Geometry: final body of the model. Coordinates: model frame, mm. Round coordinates to 2 decimals unless told otherwise and drop trailing zeros. Write each loop counter-clockwise with the first axis right and the second up, starting at its lowest first coordinate (ties: lowest second). Pieces come first, ordered by that corner, then holes. Notation, with made-up numbers: M 62,38 L 94,38 A31 ccw 94,77 Z; hole C 66,77.25 d5. An arc over 180 degrees is marked long. Use one line per item in the form item = value. Start each with the question number.
Item 1: Pin query (flat end, axial travel): pin 1 Ø5.5 at (x, z) = (46.4, 123.19) entering from +Y; pin 2 Ø7.5 at (x, z) = (102.32, 78.74) entering from +Y. Return the tip coordinate at first contact, or that it passes through.
Item 2: Ray query, probe 1 along X at (y, z) = (5.5, 123.19) (3 decimals); probe 2 along X at (y, z) = (4.25, -37.5) (3 decimals); probe 3 along X at (y, z) = (3, 78.74) (3 decimals). Return the intervals inside material, ascending.
Item 3: Section query A-A (z = 78.74). Return loops of the section in (x, y) (3 decimals).
Item 4: Section query D-D (z = 123.19). Return loops of the section in (x, y) (3 decimals), and give its area (3 significant figures).
Item 5: Section query B-B (x = 0). Return loops of the section in (y, z).
Item 6: Pull-direction query (X, two-part tool) for faces 1 (the cylindrical face through (100.39, 6.26, 76.22)), 2 (the flat face through (210.274, 6, 47)), 3 (the flat face through (44, 6, -50.8)), 4 (the flat face through (-117.475, 6, 47)); classes: pulls with the +X half, pulls with the -X half, needs draft (parallel to the pull), parting line crosses it, or undercut.
Item 7: Section query C-C (z = -38.1). Return loops of the section in (x, y) (3 decimals), and give its area (3 significant figures).
from build123d import *

# Parameters (mm, degrees)
SKETCH1_W           = 327.74935392
SKETCH1_H           = 193.04
SKETCH1_R           = 14.2875
SKETCH1_R_2         = 3.175
BOSS_EXTRUDE1_DEPTH = 12.7


with BuildPart() as part:
    # Sketch1 → Boss-Extrude1 (new body)
    with BuildSketch(Plane(origin=(0, 0, 0), x_dir=(1, 0, 0), z_dir=(0, 1, 0))):
        with Locations((46.39967696, -45.72)):
            Rectangle(SKETCH1_W, SKETCH1_H)
        with Locations(Location((0, 0, 0), (0, 0, 270))):
            Circle(SKETCH1_R, mode=Mode.SUBTRACT)
        with Locations(Location((159.47435392, -42.731024346, 0), (0, 0, 270))):
            Circle(SKETCH1_R, mode=Mode.SUBTRACT)
        with Locations(Location((-88.9, -1.817931401, 0), (0, 0, 270))):
            Circle(SKETCH1_R, mode=Mode.SUBTRACT)
        with Locations(Location((-98.425, -123.19, 0), (0, 0, 270))):
            Circle(SKETCH1_R_2, mode=Mode.SUBTRACT)
        with Locations(Location((191.22435392, -123.19, 0), (0, 0, 270))):
            Circle(SKETCH1_R_2, mode=Mode.SUBTRACT)
        with Locations(Location((191.22435392, 31.75, 0), (0, 0, 270))):
            Circle(SKETCH1_R_2, mode=Mode.SUBTRACT)
        with Locations(Location((102.32435392, -78.74, 0), (0, 0, 270))):
            Circle(SKETCH1_R_2, mode=Mode.SUBTRACT)
        with Locations(Location((46.3996786, -123.19, 0), (0, 0, 270))):
            Circle(SKETCH1_R_2, mode=Mode.SUBTRACT)
        with Locations(Location((-57.15, -25.4, 0), (0, 0, 270))):
            Circle(SKETCH1_R_2, mode=Mode.SUBTRACT)
        with Locations(Location((-104.775, 38.1, 0), (0, 0, 270))):
            Circle(SKETCH1_R_2, mode=Mode.SUBTRACT)
        with Locations(Location((51.52435392, 38.1, 0), (0, 0, 270))):
            Circle(SKETCH1_R_2, mode=Mode.SUBTRACT)
    extrude(amount=BOSS_EXTRUDE1_DEPTH)


solid = part.part
Working result:
q1.pin_1 = through
q1.pin_2 = 12.7
q2.probe_1 = -117.475 to -101.6, -95.25 to 43.225, 49.575 to 188.049, 194.399 to 210.274
q2.probe_2 = -117.475 to -107.893, -101.657 to 48.407, 54.642 to 210.274
q2.probe_3 = -117.475 to 99.149, 105.499 to 210.274
q3.outline = M -117.475,0 L 99.149,0 L 99.149,12.7 L -117.475,12.7 Z; M 105.499,0 L 210.274,0 L 210.274,12.7 L 105.499,12.7 Z
q4.outline = M -117.475,0 L -101.6,0 L -101.6,12.7 L -117.475,12.7 Z; M -95.25,0 L 43.225,0 L 43.225,12.7 L -95.25,12.7 Z; M 49.575,0 L 188.049,0 L 188.049,12.7 L 49.575,12.7 Z; M 194.399,0 L 210.274,0 L 210.274,12.7 L 194.399,12.7 Z
q4.area = 3,920 mm²
q5.outline = M 0,-50.8 L 12.7,-50.8 L 12.7,-14.29 L 0,-14.29 Z; M 0,14.29 L 12.7,14.29 L 12.7,142.24 L 0,142.24 Z
q6.face_1 = undercut
q6.face_2 = pulls with the +X half
q6.face_3 = needs draft
q6.face_4 = pulls with the -X half
q7.outline = M -117.475,0 L -107.95,0 L -107.95,12.7 L -117.475,12.7 Z; M -101.6,0 L 48.349,0 L 48.349,12.7 L -101.6,12.7 Z; M 54.699,0 L 210.274,0 L 210.274,12.7 L 54.699,12.7 Z
q7.area = 4,000 mm²
